Can you work these out from the model? Positions are in its coordinate system, mm. A direction names the side the tool comes from. Give positions to 0.01 mm unless a question says otherwise; leave off trailing zeros. Write each loop counter-clockwise with the first axis right and the second up, starting at its lowest first coordinate (ties: lowest second). Pieces come first, ordered by that corner, then holes.
from build123d import *

# Parameters (mm, degrees)
F1_DEPTH = 18


with BuildPart() as f1:
    # F0 (on Front) → F1 (new body)
    with BuildSketch(Plane.XZ):
        with BuildLine():
            Line((240.362719, 0), (280, 0))
            Line((280, 0), (352.678155, 0))
            ThreePointArc((352.678155, 0), (329.930673, 59.773689), (297.140698, 114.684155))
            Line((297.140698, 114.684155), (259.063123, 167.386681))
            ThreePointArc((259.063123, 167.386681), (249.616666, 195.090013), (257.29587, 223.334303))
            ThreePointArc((257.29587, 223.334303), (263.03537, 236.121843), (265, 250))
            Line((265, 250), (224.934809, 250))
            ThreePointArc((224.934809, 250), (202.176253, 255.479801), (184.406191, 270.718074))
            Line((184.406191, 270.718074), (91, 400))
            Line((91, 400), (84, 400))
            Line((84, 400), (84, 414))
            ThreePointArc((84, 414), (82.828427, 416.828427), (80, 418))
            Line((80, 418), (52, 418))
            ThreePointArc((52, 418), (49.171573, 416.828427), (48, 414))
            Line((48, 414), (48, 400))
            Line((48, 400), (41, 400))
            Line((41, 400), (78.778869, 336.771767))
            ThreePointArc((78.778869, 336.771767), (85.768369, 308.150895), (75.428478, 280.562962))
            ThreePointArc((75.428478, 280.562962), (67.678884, 266.146577), (65, 250))
            Line((65, 250), (102.254694, 250))
            ThreePointArc((102.254694, 250), (126.92966, 243.48731), (145.176608, 225.645844))
            Line((145.176608, 225.645844), (206.336559, 123.286094))
            ThreePointArc((206.336559, 123.286094), (231.700078, 63.947714), (240.362719, 0))
        make_face()
    extrude(amount=F1_DEPTH)


solid = f1.part
(1) Imagine slicing it at B-B, the plane x = 305.5. Write out the boundary of the cut face in (y, z), plus the area to 3 significant figures.
Returned:
outline: (-18, 0) - (0, 0) - (0, 102.61) - (-18, 102.61) - close
area: 1,850 mm2
(2) Imagine slicing it at A-A, the plane y = -12. Write out the boundary of the cut face in (x, z).
Returned:
outline: (41, 400) - (78.78, 336.77) arc R50 cw to (75.43, 280.56) arc R50 ccw to (65, 250) - (102.25, 250) arc R50 cw to (145.18, 225.65) - (206.34, 123.29) arc R240.36 cw to (240.36, 0) - (352.68, 0) arc R366.58 ccw to (297.14, 114.68) - (259.06, 167.39) arc R50 cw to (257.3, 223.33) arc R50 ccw to (265, 250) - (224.93, 250) arc R50 cw to (184.41, 270.72) - (91, 400) - (84, 400) - (84, 414) arc R4 ccw to (80, 418) - (52, 418) arc R4 ccw to (48, 414) - (48, 400) - close
(3) If I drill on L1, parallel to Z at x = 87, y = -3.25; L2, parallel to Z at x = 242, y = -13; L3, parallel to X at y = -14, z = 193, over which ranges is the centre line in solid material (lowest first)?
Returned:
L1: z = 250 to 400
L2: z = 0 to 250
L3: x = 164.68 to 249.73
(4) Will these pins go through, and if not, where does the flat tip stop? P1, Ø10, axis at x = 147.5, y = -13, coming from the -Z side; P2, Ø2, axis at y = -4, z = 138, coming from the -X side; P3, Ø1.5, axis at x = 157, y = -5, coming from the +Z side; P4, Ø2, axis at x = 241.5, z = 200, coming from the +Y side.
Returned:
P1: stops at z = 213.39
P2: stops at x = 196.95
P3: stops at z = 309.69
P4: stops at y = 0
(5) Imagine slicing it at C-C, the plane z = 159.5. Write out the boundary of the cut face in (x, y), plus the area to 3 significant figures.
Returned:
outline: (184.7, -18) - (264.76, -18) - (264.76, 0) - (184.7, 0) - close
area: 1,440 mm2
(6) For faces 1 (the face through (83, -9, 250)), 2 (the face through (185, -18, 194)), 3 (the face through (84, -9, 407)), 4 (the face through (48, -9, 407)), 5 (the face through (185, 0, 194)), which set-ups out of +Z, -Z, +X, -X, +Y, -Y let a thin tool reach every point of the face, with its end or its side?
Returned:
face 1: -Z, -X, +Y, -Y
face 2: +Z, -Z, +X, -X, -Y
face 3: +Z, +X, +Y, -Y
face 4: +Z, -X, +Y, -Y
face 5: +Z, -Z, +X, -X, +Y
(7) If we mould it in two halves opening along Z, with no side actions, what happens to faces 6 (the face through (175.33, -8.87, 175.18)), 7 (the face through (59.625, -8.874, 368.828)), 8 (the face through (66, -9, 418))? For each: +Z half, -Z half, draft (parallel to the pull), parting line (faces both ways), or undercut.
Returned:
face 6: -Z half
face 7: undercut
face 8: +Z half
